```python
from build123d import *

# Parameters (mm, degrees)
SKETCH_1_W        = 20
SKETCH_1_H        = 18
SKETCH_1_R        = 1.2
SKETCH_1_R_2      = 1.7
SKETCH_1_R_3      = 2.1
EXTRUDE_1_DEPTH   = 4
EXTRUDE_1_2_DEPTH = 4
SKETCH_2_W        = 33.123219373
SKETCH_2_H        = 12.052469136
EXTRUDE_2_DEPTH   = 1


with BuildPart() as part:
    # Sketch 1 → Extrude 1 (new body)
    with BuildSketch(Plane.XY):
        with Locations((25, 0)):
            Rectangle(SKETCH_1_W, SKETCH_1_H)
        with Locations(Location((30, -4.5, 0), (0, 0, 180))):
            Circle(SKETCH_1_R, mode=Mode.SUBTRACT)
        with Locations(Location((20, -4.5, 0), (0, 0, 180))):
            Circle(SKETCH_1_R_2, mode=Mode.SUBTRACT)
        with Locations(Location((20, 4.5, 0), (0, 0, 180))):
            Circle(SKETCH_1_R, mode=Mode.SUBTRACT)
        with Locations(Location((30, 4.5, 0), (0, 0, 180))):
            Circle(SKETCH_1_R_3, mode=Mode.SUBTRACT)
    extrude(amount=EXTRUDE_1_DEPTH)



with BuildPart() as body_2:
    # Sketch 1 → Extrude 1 2 (new body)
    with BuildSketch(Plane.XY):
        with Locations((-25, 0)):
            Rectangle(SKETCH_1_W, SKETCH_1_H)
        with Locations((-30, 4.5)):
            Circle(SKETCH_1_R_3, mode=Mode.SUBTRACT)
        with Locations((-20, 4.5)):
            Circle(SKETCH_1_R, mode=Mode.SUBTRACT)
        with Locations((-20, -4.5)):
            Circle(SKETCH_1_R_2, mode=Mode.SUBTRACT)
        with Locations((-30, -4.5)):
            Circle(SKETCH_1_R, mode=Mode.SUBTRACT)
    extrude(amount=EXTRUDE_1_2_DEPTH)


with BuildPart() as part_1:
    add(part.part)

    add(body_2.part)  # Extrude 2 merges body 2
    # Sketch 2 → Extrude 2 (add)
    with BuildSketch(Plane(origin=(0, 0, 2), x_dir=(-1, 0, 0), z_dir=(0, 0, -1))):
        with Locations((0.036443495, 0.168566002)):
            Rectangle(SKETCH_2_W, SKETCH_2_H)
    extrude(amount=EXTRUDE_2_DEPTH)


solid = part_1.part
```
CAD build for the part. Positions are in the model's coordinates, mm. A direction names the side the tool comes from. Give positions to 0.01 mm unless a question says otherwise; leave off trailing zeros. Order: outer loops, then holes, each group sorted by start corner. A loop starts at its lowest first (then second) coordinate and runs counter-clockwise, first axis right, second up.
(1) Saw through at D-D, the plane x = 20. Give the cut face in (y, z).
(2) Saw through at A-A, the plane z = 2.75. State how many separate pieces and enclosed holes the cut face has, then the cut area to 3 significant figures.
(3) Mould opens along Y. For faces 4 (the cylindrical face through (-32.1, 4.59, 1.97)), 5 (the flat face through (25, -9, 2)), 6 (the flat face through (-25, 9, 2)) say: released by +Y, released by -Y, zero draft, split by the parting line, or undercut.
(4) Saw through at B-B, the plane x = -30. Give the cut face in (y, z), then the cut area to 3 significant figures.
(5) Drill centre lines: L1, parallel to Y at x = 20, z = 2.4; L2, parallel to Y at x = -30, z = 2.85; L3, parallel to X at y = 5, z = 1.65. Where is each one in solid material? Low to high.
(6) Flat gauge pins, fed straight in: pin 1 (4 mm diameter, centred on x = -16, y = 4.5, fed in from -Z); pin 2 (0.5 mm diameter, centred on x = -4, z = 1.5, fed in from +Y); pin 3 (3 mm diameter, centred on x = -7, y = -4.5, fed in from +Z); pin 4 (6 mm diameter, centred on x = 0, y = -0.5, fed in from -Z). Where does each tip first touch, or does it go through?
(7) Saw through at C-C, the plane y = -4.5. Give the cut face in (x, z).
(8) Tool access for faces 1 (the flat face through (0, 0, 1)), 2 (the cylindrical face through (-21.2, 4.55, 1.97)), 3 (the flat face through (0, 0, 2)): list every direction of +Z, -Z, +X, -X, +Y, -Y with a clear straight run to the whole face (end or side of a thin tool).
Results found:
1. outline: (-9, 0) - (-6.2, 0) - (-6.2, 4) - (-9, 4) - close; (-2.8, 0) - (3.3, 0) - (3.3, 4) - (-2.8, 4) - close; (5.7, 0) - (9, 0) - (9, 4) - (5.7, 4) - close
2. separate pieces: 2
2. enclosed holes: 8
2. area: 656 mm2
3. face 4: undercut
3. face 5: released by -Y
3. face 6: released by +Y
4. outline: (-9, 0) - (-5.7, 0) - (-5.7, 4) - (-9, 4) - close; (-3.3, 0) - (2.4, 0) - (2.4, 4) - (-3.3, 4) - close; (6.6, 0) - (9, 0) - (9, 4) - (6.6, 4) - close
4. area: 45.6 mm2
5. L1: y = -9 to -6.2, -2.8 to 3.3, 5.7 to 9
5. L2: y = -9 to -5.7, -3.3 to 2.4, 6.6 to 9
5. L3: x = -35 to -32.04, -27.96 to -21.09, -18.91 to 18.91, 21.09 to 27.96, 32.04 to 35
6. pin 1: stops at z = 0
6. pin 2: stops at y = 6.19
6. pin 3: stops at z = 2
6. pin 4: stops at z = 1
7. outline: (-35, 0) - (-31.2, 0) - (-31.2, 4) - (-35, 4) - close; (-28.8, 0) - (-21.7, 0) - (-21.7, 4) - (-28.8, 4) - close; (-18.3, 0) - (-15, 0) - (-15, 1) - (15, 1) - (15, 0) - (18.3, 0) - (18.3, 4) - (15, 4) - (15, 2) - (-15, 2) - (-15, 4) - (-18.3, 4) - close; (21.7, 0) - (28.8, 0) - (28.8, 4) - (21.7, 4) - close; (31.2, 0) - (35, 0) - (35, 4) - (31.2, 4) - close
8. face 1: -Z, +Y, -Y
8. face 2: +Z, -Z
8. face 3: +Z, +Y, -Y
